from build123d import *

# Parameters (mm, degrees)
RESSALTO_EXTRUS_O1_DEPTH = 285


with BuildPart() as part:
    # Esboço1 → Ressalto-extrusão1 (new body)
    with BuildSketch(Plane.XY):
        with BuildLine():
            Line((0, 0), (-121.6, 0))
            Line((-121.6, 0), (-121.6, 6.35))
            Line((-121.6, 6.35), (-119.6, 6.35))
            Line((-119.6, 6.35), (-119.6, 4))
            Line((-119.6, 4), (-111.6, 4))
            Line((-111.6, 4), (-111.6, 14))
            Line((-111.6, 14), (-119.6, 14))
            Line((-119.6, 14), (-119.6, 11.65))
            Line((-119.6, 11.65), (-121.6, 11.65))
            Line((-121.6, 11.65), (-121.6, 65.055990081))
            ThreePointArc((-121.6, 65.055990081), (-121.94756763, 65.895092566), (-122.786670115, 66.242660196))
            Line((-122.786670115, 66.242660196), (-133.65, 66.242660196))
            Line((-133.65, 66.242660196), (-133.65, 69))
            Line((-133.65, 69), (-122.786670115, 69))
            ThreePointArc((-122.786670115, 69), (-119.997833956, 67.84482624), (-118.842660196, 65.055990081))
            Line((-118.842660196, 65.055990081), (-117.547286109, 27))
            ThreePointArc((-117.547286109, 27), (-112.847286109, 22.3), (-108.147286109, 27))
            Line((-108.147286109, 27), (-106.75, 68.05))
            ThreePointArc((-106.75, 68.05), (-105.8, 69), (-104.85, 68.05))
            Line((-104.85, 68.05), (-103, 13.7))
            ThreePointArc((-103, 13.7), (-98.3, 9), (-93.6, 13.7))
            Line((-93.6, 13.7), (-91.75, 68.05))
            ThreePointArc((-91.75, 68.05), (-90.8, 69), (-89.85, 68.05))
            Line((-89.85, 68.05), (-88, 13.7))
            ThreePointArc((-88, 13.7), (-83.3, 9), (-78.6, 13.7))
            Line((-78.6, 13.7), (-76.75, 68.05))
            ThreePointArc((-76.75, 68.05), (-75.8, 69), (-74.85, 68.05))
            Line((-74.85, 68.05), (-73, 13.7))
            ThreePointArc((-73, 13.7), (-68.3, 9), (-63.6, 13.7))
            Line((-63.6, 13.7), (-61.75, 68.05))
            ThreePointArc((-61.75, 68.05), (-60.8, 69), (-59.85, 68.05))
            Line((-59.85, 68.05), (-58, 13.7))
            ThreePointArc((-58, 13.7), (-53.3, 9), (-48.6, 13.7))
            Line((-48.6, 13.7), (-46.75, 68.05))
            ThreePointArc((-46.75, 68.05), (-45.8, 69), (-44.85, 68.05))
            Line((-44.85, 68.05), (-43, 13.7))
            ThreePointArc((-43, 13.7), (-38.3, 9), (-33.6, 13.7))
            Line((-33.6, 13.7), (-31.75, 68.05))
            ThreePointArc((-31.75, 68.05), (-30.8, 69), (-29.85, 68.05))
            Line((-29.85, 68.05), (-28, 13.7))
            ThreePointArc((-28, 13.7), (-23.3, 9), (-18.6, 13.7))
            Line((-18.6, 13.7), (-16.75, 68.05))
            ThreePointArc((-16.75, 68.05), (-15.8, 69), (-14.85, 68.05))
            Line((-14.85, 68.05), (-13.452713891, 27))
            ThreePointArc((-13.452713891, 27), (-8.752713891, 22.3), (-4.052713891, 27))
            Line((-4.052713891, 27), (-2.757339804, 65.055990081))
            ThreePointArc((-2.757339804, 65.055990081), (-1.602166044, 67.84482624), (1.186670115, 69))
            Line((1.186670115, 69), (12.05, 69))
            Line((12.05, 69), (12.05, 66.242660196))
            Line((12.05, 66.242660196), (1.186670115, 66.242660196))
            ThreePointArc((1.186670115, 66.242660196), (0.34756763, 65.895092566), (0, 65.055990081))
            Line((0, 65.055990081), (0, 11.65))
            Line((0, 11.65), (-2, 11.65))
            Line((-2, 11.65), (-2, 14))
            Line((-2, 14), (-10, 14))
            Line((-10, 14), (-10, 4))
            Line((-10, 4), (-2, 4))
            Line((-2, 4), (-2, 6.35))
            Line((-2, 6.35), (0, 6.35))
            Line((0, 6.35), (0, 0))
        make_face()
    extrude(amount=RESSALTO_EXTRUS_O1_DEPTH)


solid = part.part
Read the model definition and answer for the solid it produces. Units are mm, in the model's axes. A direction names the side the tool comes from. Round coordinates to 2 decimals unless told otherwise and drop trailing zeros. Order: outer loops, then holes, each group sorted by start corner. A loop starts at its lowest first (then second) coordinate and runs counter-clockwise, first axis right, second up.
1) Straight lines are drawn through the part: L1, parallel to Y at x = -127, z = 227.5; L2, parallel to Y at x = -112, z = 78.5; L3, parallel to Y at x = -16, z = 210.5. For each, find the intervals that lie inside material, in ascending order.
2) The mould has two halves that part along Y. Classify faces 3 (the face through (-83.4, 9, 140.5)), 4 (the face through (-111.6, 9, 141)), 5 (the face through (-60, 0, 141)): released by +Y, released by -Y, zero draft, split by the parting line, or undercut.
3) The part is cut by section B-B on y = 53.5. Give the number of separate pieces and of enclosed holes in the cut face, plus the area to 3 significant figures.
4) For faces 1 (the face through (-8.86, 22.3, 140.5)), 2 (the face through (-6, 4, 141)), determine the directions among +Z, -Z, +X, -X, +Y, -Y from which every point of the face is accessible in a straight line to the end or side of a thin tool.
5) The part is cut by section A-A on x = -53.3. Write down the section's boundary in (y, z), plus the area to 4 significant figures.
6) Flat-ended cylindrical pins translate along their axes: pin 1 (8.5 mm diameter, centred on x = 9, z = 102.5, fed in from -Y); pin 2 (0.6 mm diameter, centred on x = -120.5, z = 202, fed in from -Y); pin 3 (3 mm diameter, centred on y = 9.5, z = 85.5, fed in from +X); pin 4 (2.5 mm diameter, centred on y = 5.5, z = 198.5, fed in from +X). Find the tip coordinate at first contact, or state that the pin passes through.
Resolved:
1. L1: y = 66.24 to 69
1. L2: y = 0 to 4, 14 to 22.38
1. L3: y = 0 to 68.98
2. face 3: released by +Y
2. face 4: undercut
2. face 5: released by -Y
3. separate pieces: 9
3. enclosed holes: 0
3. area: 7,560 mm2
4. face 1: +Z, -Z, +Y
4. face 2: +Z, -Z
5. outline: (0, 0) - (9, 0) - (9, 285) - (0, 285) - close
5. area: 2,565 mm2
6. pin 1: stops at y = 66.24
6. pin 2: stops at y = 0
6. pin 3: stops at x = -10
6. pin 4: stops at x = 0
